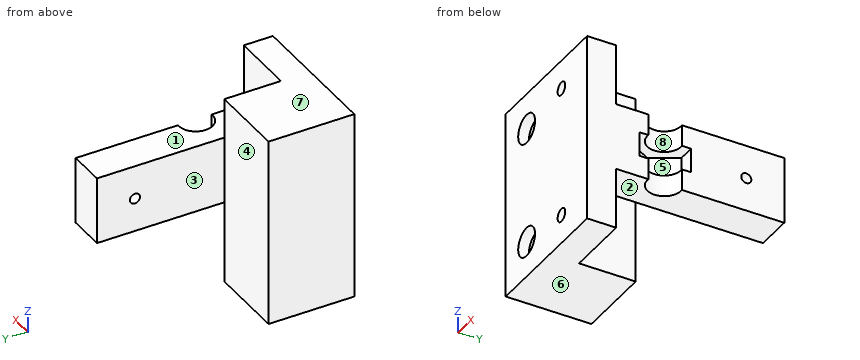
```python
from build123d import *

# Parameters (mm, degrees)
SKETCH_1_W          = 23
SKETCH_1_H          = 64.4
EXTRUDE_1_DEPTH     = 8
SKETCH_3_W          = 23
SKETCH_3_H          = 64.4
SKETCH_3_R          = 5.5
EXTRUDE_2_DEPTH     = 7
SKETCH_4_W          = 23
SKETCH_4_H          = 64.4
SKETCH_4_R          = 5.5
EXTRUDE_3_DEPTH     = 7
SKETCH_5_R          = 1.65
CUT_EXTRUDE_1_DEPTH = 24
SKETCH_6_W          = 22
SKETCH_6_H          = 64.4
CUT_EXTRUDE_2_DEPTH = 11
EXTRUDE_4_DEPTH     = 9.5
SKETCH_8_R          = 2.15
CUT_EXTRUDE_3_DEPTH = 10.5
SKETCH_9_R          = 4.75
CUT_EXTRUDE_4_DEPTH = 3.5
SKETCH_10_W         = 25
SKETCH_10_H         = 62
EXTRUDE_5_DEPTH     = 18.5


with BuildPart() as part:
    # 草圖1 → 填料-伸長1 (new body)
    with BuildSketch(Plane.XY):
        with Locations((-0.36746988, -27.579314659)):
            Rectangle(SKETCH_1_W, SKETCH_1_H)
        Polygon((9.38974967, -34.279314659), (4.511139895, -25.829314659), (-5.246079654, -25.829314659), (-10.124689429, -34.279314659), (-5.246079654, -42.729314659), (4.511139895, -42.729314659), align=None, mode=Mode.SUBTRACT)
    extrude(amount=EXTRUDE_1_DEPTH)

    # 草圖3 → 填料-伸長2 (add)
    with BuildSketch(Plane.XY.offset(8)):
        with Locations((-0.36746988, -27.579314659)):
            Rectangle(SKETCH_3_W, SKETCH_3_H)
        with Locations((-0.36746988, -34.279314659)):
            Circle(SKETCH_3_R, mode=Mode.SUBTRACT)
    extrude(amount=EXTRUDE_2_DEPTH)

    # 草圖4 → 填料-伸長3 (add)
    with BuildSketch(Plane(origin=(0, 0, 0), x_dir=(-1, 0, 0), z_dir=(0, 0, -1))):
        with Locations((0.36746988, -27.579314659)):
            Rectangle(SKETCH_4_W, SKETCH_4_H)
        with Locations((0.36746988, -34.279314659)):
            Circle(SKETCH_4_R, mode=Mode.SUBTRACT)
    extrude(amount=EXTRUDE_3_DEPTH)

    # 草圖5 → 除料-伸長1 (cut, through all)
    with BuildSketch(Plane(origin=(11.13253012, 0, 0), x_dir=(0, 0, -1), z_dir=(1, 0, 0))):
        with Locations((-4, -7.779314659)):
            Circle(SKETCH_5_R)
    extrude(amount=-CUT_EXTRUDE_1_DEPTH, mode=Mode.SUBTRACT)

    # 草圖6 → 除料-伸長2 (cut)
    with BuildSketch(Plane(origin=(11.13253012, 0, 0), x_dir=(0, 0, -1), z_dir=(1, 0, 0))):
        with Locations((-4, -27.579314659)):
            Rectangle(SKETCH_6_W, SKETCH_6_H)
    extrude(amount=-CUT_EXTRUDE_2_DEPTH, mode=Mode.SUBTRACT)

    # 草圖7 → 填料-伸長4 (add)
    with BuildSketch(Plane.XZ.offset(59.779314659)):
        Polygon((0.13253012, 15), (0.13253012, 35), (-45.86746988, 35), (-45.86746988, -27), (0.13253012, -27), (0.13253012, -7), align=None)
    extrude(amount=-EXTRUDE_4_DEPTH)

    # 草圖8 → 除料-伸長3 (cut, through all)
    with BuildSketch(Plane(origin=(0, -50.279314659, 0), x_dir=(1, 0, 0), z_dir=(0, 1, 0))):
        with Locations((-14.36746988, 17.5)):
            Circle(SKETCH_8_R)
        with Locations((-14.36746988, -25.5)):
            Circle(SKETCH_8_R)
    extrude(amount=-CUT_EXTRUDE_3_DEPTH, mode=Mode.SUBTRACT)

    # 草圖9 → 除料-伸長4 (cut)
    with BuildSketch(Plane.XZ.offset(59.779314659)):
        with Locations((-34.06746988, 23.2)):
            Circle(SKETCH_9_R)
        with Locations((-34.06746988, -15.2)):
            Circle(SKETCH_9_R)
    extrude(amount=-CUT_EXTRUDE_4_DEPTH, mode=Mode.SUBTRACT)

    # 草圖10 → 填料-伸長5 (add)
    with BuildSketch(Plane(origin=(0, -50.279314659, 0), x_dir=(1, 0, 0), z_dir=(0, 1, 0))):
        with Locations((-33.36746988, -4)):
            Rectangle(SKETCH_10_W, SKETCH_10_H)
    extrude(amount=EXTRUDE_5_DEPTH)


solid = part.part
```
The listing builds one solid part. Answer for the finished solid, in the listing's coordinates (mm). Face numbers are marked on the shaded views. A direction names the side the tool comes from. Coordinates: 2 decimals unless noted, no trailing zeros. Loops run counter-clockwise (first coordinate to the right, second up) from the corner with the lowest first, then second, coordinate; pieces in that order, holes last. Notation, with made-up numbers: M 82,40 L 136,40 A24 cw 136,65 Z; hole C -16.5,7 d6. An arc over 180 degrees is marked long. Answer as a JSON object with one key per item and string values. Group by question number.
Item 1: Section D-D (z = 4) is taken. Write down the section's boundary in (x, y).
Item 2: Determine the mould class of the marked faces 5, 6, 7 and 8 for opening direction Z: +Z half, -Z half, draft (parallel to the pull), parting line (faces both ways), or undercut.
Item 3: Section A-A (z = -17.5) is taken. Write down the section's boundary in (x, y), and give its area (3 significant figures).
Item 4: Section C-C (x = -25) is taken. Write down the section's boundary in (y, z).
Item 5: Consider L1, parallel to Y at x = -3, z = 4; L2, parallel to X at y = -50, z = 10; L3, parallel to X at y = -58, z = -17. Determine where each line is inside the solid, lowest interval first.
Item 6: Each of these flat-tipped pins is pushed along its axis until it touches: P1, Ø20.5, axis at y = -38.5, z = -5, coming from the +X side; P2, Ø10, axis at x = -0.37, y = -34.28, coming from the -Z side; P3, Ø3, axis at x = -6, y = -31, coming from the +Z side; P4, Ø5, axis at x = -23, z = 0.5, coming from the +Y side. Where does it stop, or does it pass through?
Item 7: Section B-B (y = -46) is taken. Write down the section's boundary in (x, z).
Item 8: Which of the six approach directions +Z, -Z, +X, -X, +Y, -Y give full straight-line access (tool end or side, diameter ignored) to the marked faces 1, 2, 3 and 4?
Solved:
{
 "1": {"outline": "M -45.87,-59.78 L 0.13,-59.78 L 0.13,-42.73 L -5.25,-42.73 L -10.12,-34.28 L -5.25,-25.83 L 0.13,-25.83 L 0.13,-9.43 L -11.87,-9.43 L -11.87,-50.28 L -20.87,-50.28 L -20.87,-31.78 L -45.87,-31.78 Z; M -11.87,-6.13 L 0.13,-6.13 L 0.13,4.62 L -11.87,4.62 Z"},
 "2": {"face 5": "undercut", "face 6": "-Z half", "face 7": "+Z half", "face 8": "draft"},
 "3": {"outline": "M -45.87,-59.78 L -38.22,-59.78 L -38.22,-56.28 L -29.91,-56.28 L -29.91,-59.78 L -16.52,-59.78 L -16.52,-50.28 L -20.87,-50.28 L -20.87,-31.78 L -45.87,-31.78 Z; M -12.22,-59.78 L 0.13,-59.78 L 0.13,-50.28 L -12.22,-50.28 Z", "area": "830 mm2"},
 "4": {"outline": "M -59.78,-27 L -31.78,-27 L -31.78,35 L -59.78,35 Z"},
 "5": {"L1": "y = -59.78 to -42.73, -25.83 to -9.43, -6.13 to 4.62", "L2": "x = -45.87 to -20.87, -11.87 to 0.13", "L3": "x = -45.87 to -38.46, -29.67 to -16.46, -12.28 to 0.13"},
 "6": {"P1": "stops at x = 0.13", "P2": "passes through", "P3": "stops at z = 15", "P4": "stops at y = -31.78"},
 "7": {"outline": "M -45.87,-27 L -20.87,-27 L -20.87,35 L -45.87,35 Z; M -11.87,-7 L 0.13,-7 L 0.13,15 L -11.87,15 Z"},
 "8": {"face 1": "+Z, +X, +Y", "face 2": "-Z, +X, +Y", "face 3": "+Z, -Z, +Y", "face 4": "+Z, -Z, -X, +Y"}
}
